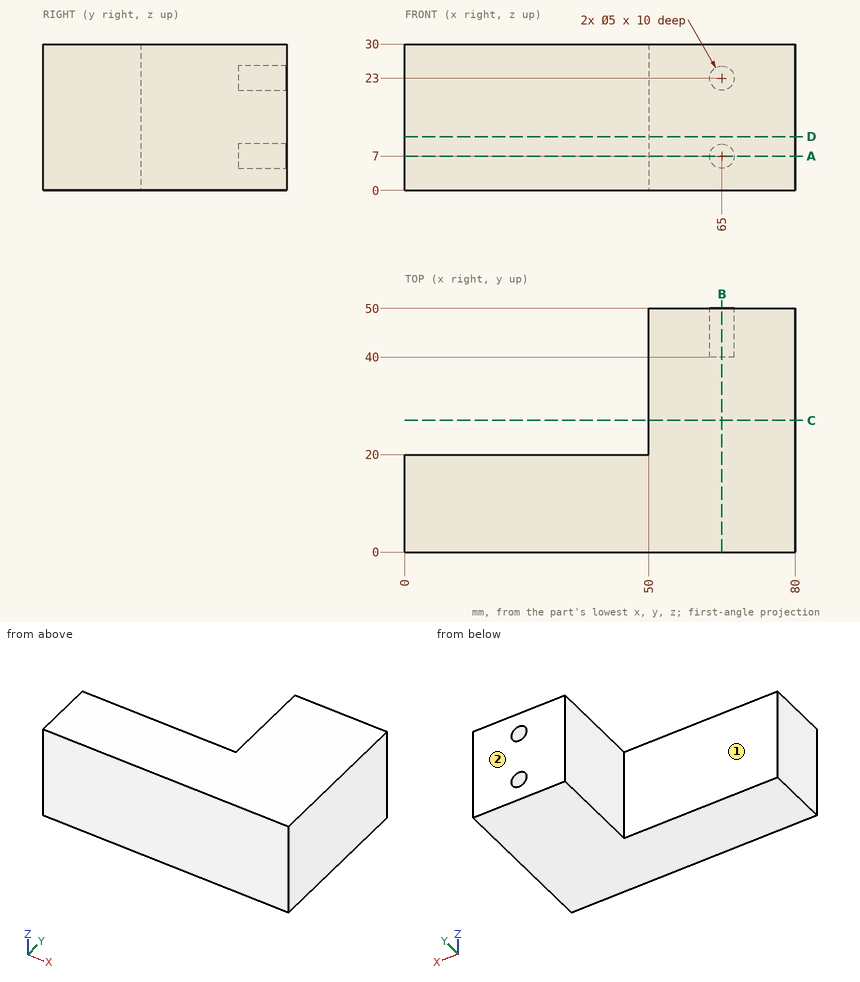
Input: dimensioned drawing with shaded views. Units: mm. Origin: part minimum x, y, z. A direction names the side the tool comes from. Coordinates: 2 decimals unless noted, no trailing zeros. Order: outer loops, then holes, each group sorted by start corner. A loop starts at its lowest first (then second) coordinate and runs counter-clockwise, first axis right, second up.
1. Access query for the marked faces 1 and 2. Directions: +Z, -Z, +X, -X, +Y, -Y. A direction counts if a zero-diameter tool reaches every point of the face in a straight line with its end or side. Return the directions, or none.
Checked values:
face 1: +Z, -Z, -X, +Y
face 2: +Z, -Z, +X, -X, +Y
2. Cut plane B-B, the plane x = 65. Return loops of the section in (y, z), plus the area to 3 significant figures.
Checked values:
outline: (0, 0) - (50, 0) - (50, 4.5) - (40, 4.5) - (40, 9.5) - (50, 9.5) - (50, 20.5) - (40, 20.5) - (40, 25.5) - (50, 25.5) - (50, 30) - (0, 30) - close
area: 1,400 mm2
3. Cut plane A-A, the plane z = 7. Return loops of the section in (x, y), plus the area to 3 significant figures.
Checked values:
outline: (0, 0) - (80, 0) - (80, 50) - (67.5, 50) - (67.5, 40) - (62.5, 40) - (62.5, 50) - (50, 50) - (50, 20) - (0, 20) - close
area: 2,450 mm2
4. Contact query for flat-ended pins moving along their axis: P1, Ø4, axis at x = 65, z = 23, coming from the +Y side; P2, Ø1, axis at y = 26, z = 25, coming from the -X side; P3, Ø5, axis at x = 17, z = 10.5, coming from the +Y side. Output: stop coordinate, or through.
Checked values:
P1: stops at y = 40
P2: stops at x = 50
P3: stops at y = 20
5. Ray query, line 1 along X through (y, z) = (47, 7); line 2 along Y through (x, z) = (7.5, 22); line 3 along X through (y, z) = (24, 6.25). Return the intervals inside material, ascending.
Checked values:
line 1: x = 50 to 62.5, 67.5 to 80
line 2: y = 0 to 20
line 3: x = 50 to 80
6. Cut plane D-D, the plane z = 11. Return loops of the section in (x, y).
Checked values:
outline: (0, 0) - (80, 0) - (80, 50) - (50, 50) - (50, 20) - (0, 20) - close
7. Cut plane C-C, the plane y = 27. Return loops of the section in (x, z).
Checked values:
outline: (50, 0) - (80, 0) - (80, 30) - (50, 30) - close
